For this review, use the dimensioned drawing (mm, ordinates from the lowest corner) and the shaded views. Round coordinates to 2 decimals unless told otherwise and drop trailing zeros. Write each loop counter-clockwise with the first axis right and the second up, starting at its lowest first coordinate (ties: lowest second). Pieces come first, ordered by that corner, then holes. Notation, with made-up numbers: M 80,60.25 L 94,60.25 A15 ccw 94,83.25 Z; hole C -31.75,-40 d1. An arc over 180 degrees is marked long. Answer in a Markdown table with one row per item.
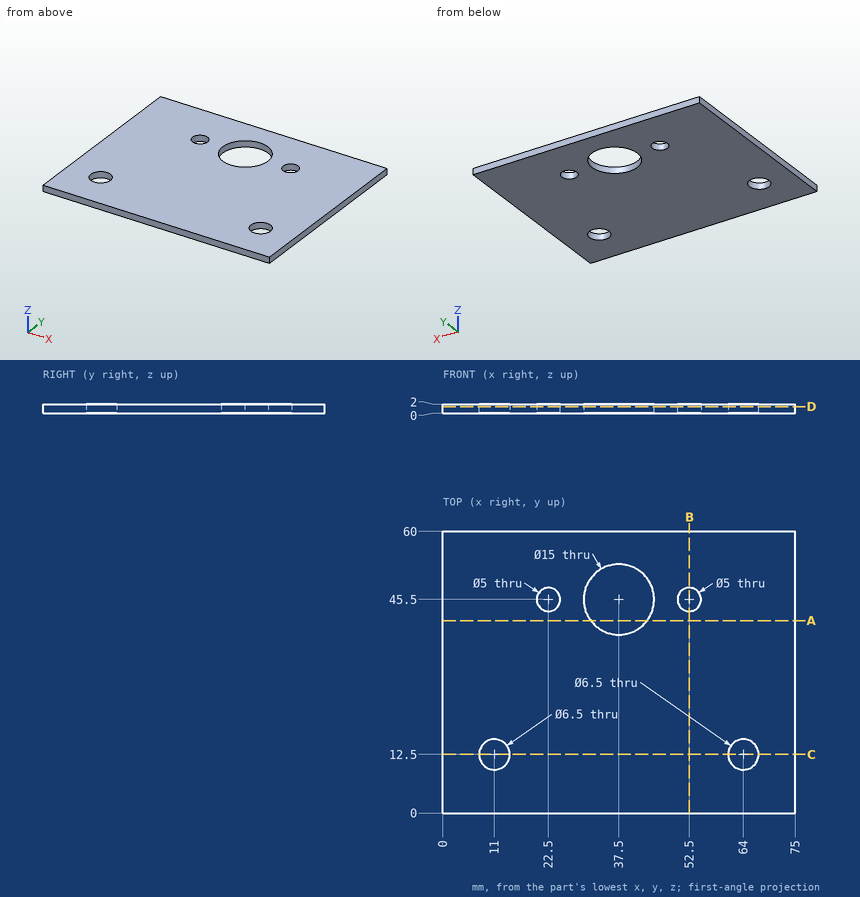
Q1. Take a section at A-A (y = 41). State the section outline as (x, z) points.
Found:
| item | result |
|---|---|
| outline | M 0,0 L 31.5,0 L 31.5,2 L 0,2 Z; M 43.5,0 L 75,0 L 75,2 L 43.5,2 Z |
Q2. Take a section at B-B (x = 52.5). State the section outline as (y, z) points.
Found:
| item | result |
|---|---|
| outline | M 0,0 L 43,0 L 43,2 L 0,2 Z; M 48,0 L 60,0 L 60,2 L 48,2 Z |
Q3. Take a section at D-D (z = 1.45). State the section outline as (x, y) points, then the cut area to 3 significant figures.
Found:
| item | result |
|---|---|
| outline | M 0,0 L 75,0 L 75,60 L 0,60 Z; hole C 11,12.5 d6.5; hole C 22.5,45.5 d5; hole C 37.5,45.5 d15; hole C 52.5,45.5 d5; hole C 64,12.5 d6.5 |
| area | 4,220 mm² |
Q4. For probe 1 along Y at (x, z) = (22.5, 0.9); probe 2 along Y at (x, z) = (64, 1.1); probe 3 along X at (y, z) = (43.5, 0.7), list the stretches that pass through material, from the lowest coordinate up.
Found:
| item | result |
|---|---|
| probe 1 | 0 to 43, 48 to 60 |
| probe 2 | 0 to 9.25, 15.75 to 60 |
| probe 3 | 0 to 21, 24 to 30.27, 44.73 to 51, 54 to 75 |
Q5. Take a section at C-C (y = 12.5). State the section outline as (x, z) points.
Found:
| item | result |
|---|---|
| outline | M 0,0 L 7.75,0 L 7.75,2 L 0,2 Z; M 14.25,0 L 60.75,0 L 60.75,2 L 14.25,2 Z; M 67.25,0 L 75,0 L 75,2 L 67.25,2 Z |
